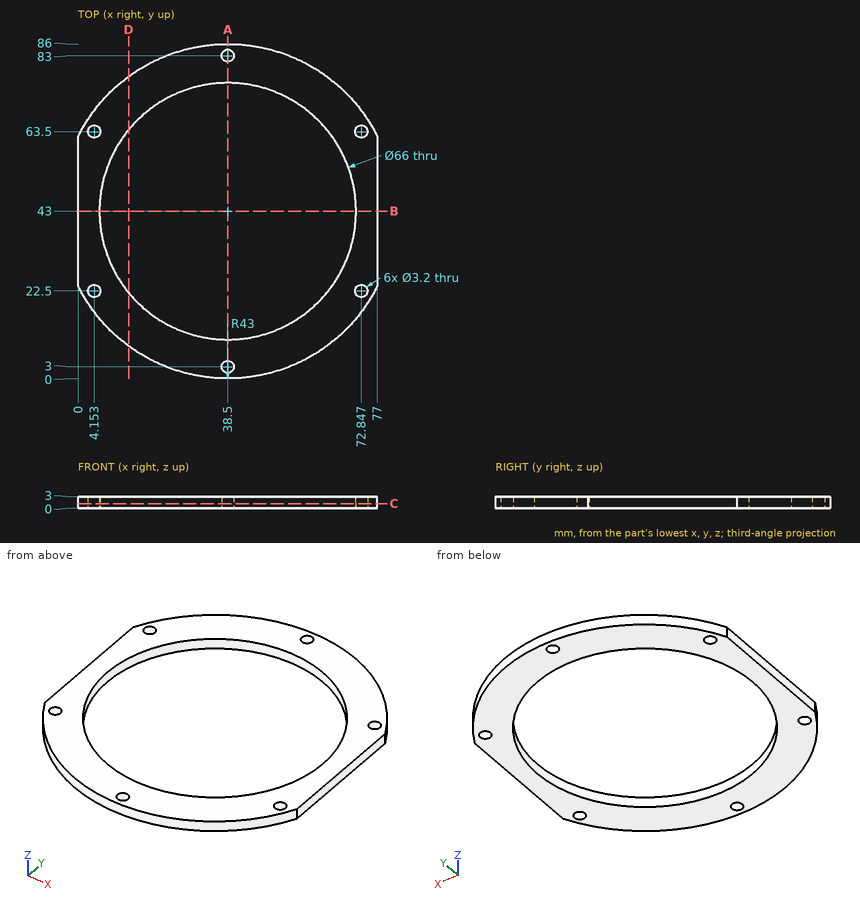
Geometry check sheet. Reference: drawing and pictorial views, mm from the part's lowest x, y, z. Round coordinates to 2 decimals unless told otherwise and drop trailing zeros. Loops run counter-clockwise (first coordinate to the right, second up) from the corner with the lowest first, then second, coordinate; pieces in that order, holes last. Notation, with made-up numbers: M 3.5,76 L 24.5,76 A22 cw 24.5,110 Z; hole C 27,25 d9. An arc over 180 degrees is marked long. One line per item, written item: value.
(1) Sectioned sample at C-C, the plane z = 1.15. Record the cut outline in (x, y), then the cut area to 3 significant figures.
Computed values:
outline: M 0,23.85 A43 ccw 77,23.85 L 77,62.15 A43 ccw 0,62.15 Z; hole C 4.15,22.5 d3.2; hole C 4.15,63.5 d3.2; hole C 38.5,43 d66; hole C 38.5,3 d3.2; hole C 38.5,83 d3.2; hole C 72.85,22.5 d3.2; hole C 72.85,63.5 d3.2
area: 2,110 mm^2
(2) Sectioned sample at A-A, the plane x = 38.5. Record the cut outline in (y, z).
Computed values:
outline: M 0,0 L 1.4,0 L 1.4,3 L 0,3 Z; M 4.6,0 L 10,0 L 10,3 L 4.6,3 Z; M 76,0 L 81.4,0 L 81.4,3 L 76,3 Z; M 84.6,0 L 86,0 L 86,3 L 84.6,3 Z
(3) Thickness scan on line 1 (Y direction, x = 38.5, z = 2.15); line 2 (Y direction, x = 38, z = 0.65) (1 decimal); line 3 (Y direction, x = 50.5, z = 1.05). Record the ranges inside material, lowest first.
Computed values:
line 1: y = 0 to 1.4, 4.6 to 10, 76 to 81.4, 84.6 to 86
line 2: y = 0 to 1.5, 4.5 to 10, 76 to 81.5, 84.5 to 86
line 3: y = 1.71 to 12.26, 73.74 to 84.29
(4) Sectioned sample at B-B, the plane y = 43. Record the cut outline in (x, z), then the cut area to 3 significant figures.
Computed values:
outline: M 0,0 L 5.5,0 L 5.5,3 L 0,3 Z; M 71.5,0 L 77,0 L 77,3 L 71.5,3 Z
area: 33.0 mm^2
(5) Sectioned sample at D-D, the plane x = 13. Record the cut outline in (y, z).
Computed values:
outline: M 8.38,0 L 22.05,0 L 22.05,3 L 8.38,3 Z; M 63.95,0 L 77.62,0 L 77.62,3 L 63.95,3 Z
(6) Depth check by flat-ended pin: pin 1 Ø1 at (x, z) = (27.5, 0.5) entering from +Y; pin 2 Ø1 at (y, z) = (10, 2.5) entering from +X (1 decimal). Enter the tip coordinate at first touch or a pass-through.
Computed values:
pin 1: stops at y = 84.7
pin 2: stops at x = 66.7
